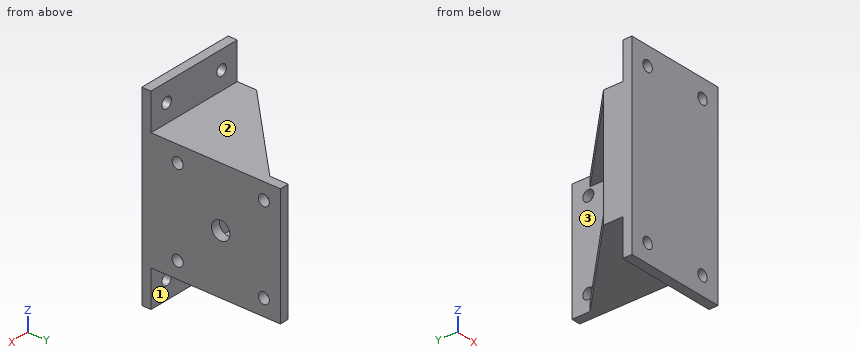
from build123d import *

# Parameters (mm, degrees)
BOSS_EXTRUDE1_DEPTH = 65
BOSS_EXTRUDE2_DEPTH = 5
BOSS_EXTRUDE3_DEPTH = 5
SKETCH4_R           = 5
SKETCH4_R_2         = 3
CUT_EXTRUDE1_DEPTH  = 102.612007165
SKETCH5_W           = 55
SKETCH5_H           = 20
BOSS_EXTRUDE4_DEPTH = 5
SKETCH6_R           = 3
CUT_EXTRUDE2_DEPTH  = 5


with BuildPart() as part:
    # Sketch1 → Boss-Extrude1 (new body)
    with BuildSketch(Plane.XY):
        Polygon((0, 0), (0, 60), (5, 60), (5, -15.5), (-50, -15.5), (-50, 0), align=None)
    extrude(amount=BOSS_EXTRUDE1_DEPTH)

    # Sketch2 → Boss-Extrude2 (add)
    with BuildSketch(Plane(origin=(0, 0, 0), x_dir=(-1, 0, 0), z_dir=(0, 0, -1))):
        Polygon((0, 0), (50, 0), (0, 50), align=None)
    extrude(amount=-BOSS_EXTRUDE2_DEPTH)

    # Sketch3 → Boss-Extrude3 (add)
    with BuildSketch(Plane.XY.offset(65)):
        Polygon((-50, 0), (0, 0), (0, 50), align=None)
    extrude(amount=-BOSS_EXTRUDE3_DEPTH)

    # Sketch4 → Cut-Extrude1 (cut, through all)
    with BuildSketch(Plane.ZY):
        with Locations(Location((32.5, 27.5, 0), (0, 0, 270))):
            Circle(SKETCH4_R)
        with Locations(Location((9, 51, 0), (0, 0, 270))):
            Circle(SKETCH4_R_2)
        with Locations(Location((56, 51, 0), (0, 0, 270))):
            Circle(SKETCH4_R_2)
        with Locations(Location((56, 4, 0), (0, 0, 270))):
            Circle(SKETCH4_R_2)
        with Locations(Location((9, 4, 0), (0, 0, 270))):
            Circle(SKETCH4_R_2)
    extrude(amount=-CUT_EXTRUDE1_DEPTH, mode=Mode.SUBTRACT)

    # Sketch5 → Boss-Extrude4 (add)
    with BuildSketch(Plane.XZ.offset(15.5)):
        with Locations((-22.5, -10)):
            Rectangle(SKETCH5_W, SKETCH5_H)
        with Locations((-22.5, 75)):
            Rectangle(SKETCH5_W, SKETCH5_H)
    extrude(amount=-BOSS_EXTRUDE4_DEPTH)

    # Sketch6 → Cut-Extrude2 (cut)
    with BuildSketch(Plane(origin=(0, -10.5, 0), x_dir=(1, 0, 0), z_dir=(0, 1, 0))):
        with Locations(Location((-5, 10, 0), (0, 0, 180))):
            Circle(SKETCH6_R)
        with Locations(Location((-40, 10, 0), (0, 0, 180))):
            Circle(SKETCH6_R)
        with Locations((-5, -75)):
            Circle(SKETCH6_R)
        with Locations((-40, -75)):
            Circle(SKETCH6_R)
    extrude(amount=-CUT_EXTRUDE2_DEPTH, mode=Mode.SUBTRACT)


solid = part.part
Model file for the job. Use its own axes, mm. Face numbers are marked on the shaded views. A direction names the side the tool comes from. Give positions to 0.01 mm unless a question says otherwise; leave off trailing zeros. Write each loop counter-clockwise with the first axis right and the second up, starting at its lowest first coordinate (ties: lowest second). Pieces come first, ordered by that corner, then holes. Notation, with made-up numbers: (10.25, 52) - (54.25, 52) arc R15 ccw to (54.25, 78) - close; hole circle Ø7 at (-35, -28). An arc over 180 degrees is marked (long way). Answer as CSV lines item,"result".
1. Pin check, flat tips, straight feed: pin 1 (25 mm diameter, centred on x = -19.5, y = 35.5, fed in from +Z); pin 2 (6 mm diameter, centred on x = -34.5, z = -9.5, fed in from +Y); pin 3 (6 mm diameter, centred on x = -38.5, z = 36.5, fed in from +Y). Stop position of each tip, or through.
Responses:
pin 1,"stops at z = 65"
pin 2,"stops at y = -10.5"
pin 3,"stops at y = 0"
2. Band-saw the part on D-D (y = 4). Write the cut outline in (x, z).
Responses:
outline,"(-46, 0) - (5, 0) - (5, 6) - (0, 6) - (0, 5) - (-46, 5) - close; (-46, 60) - (0, 60) - (0, 59) - (5, 59) - (5, 65) - (-46, 65) - close; (0, 12) - (5, 12) - (5, 53) - (0, 53) - close"
3. Band-saw the part on C-C (x = -11.5). Write the cut outline in (y, z).
Responses:
outline,"(-15.5, -20) - (-10.5, -20) - (-10.5, 0) - (38.5, 0) - (38.5, 5) - (0, 5) - (0, 60) - (38.5, 60) - (38.5, 65) - (-10.5, 65) - (-10.5, 85) - (-15.5, 85) - close"
4. Drill centre lines: L1, parallel to Z at x = -5, y = -13.45; L2, parallel to Z at x = 3, y = 4; L3, parallel to X at y = -12.05, z = 75. Where is each one in solid material? Low to high. Write a range as [from, to].
Responses:
L1,"z = [-20, -13], [-7, 72], [78, 85]"
L2,"z = [0, 6], [12, 53], [59, 65]"
L3,"x = [-50, -43], [-37, -8], [-2, 5]"
5. Band-saw the part on B-B (y = 27.5). Write the cut outline in (x, z), and give its area (3 significant figures).
Responses:
outline,"(-22.5, 0) - (5, 0) - (5, 27.5) - (0, 27.5) - (0, 5) - (-22.5, 5) - close; (-22.5, 60) - (0, 60) - (0, 37.5) - (5, 37.5) - (5, 65) - (-22.5, 65) - close"
area,"500 mm2"
6. Band-saw the part on A-A (z = 9). Write the cut outline in (x, y).
Responses:
outline,"(-50, -15.5) - (5, -15.5) - (5, 1) - (0, 1) - (0, 0) - (-50, 0) - close; (0, 7) - (5, 7) - (5, 48) - (0, 48) - close; (0, 54) - (5, 54) - (5, 60) - (0, 60) - close"
7. 3-axis set-ups, long thin cutter, end or side, ignore diameter. For the marked faces 1, 2 and 3: which of +Z, -Z, +X, -X, +Y, -Y reach the whole face in a straight line?
Responses:
face 1,"-Z, +X, -X, +Y"
face 2,"+Z, +X, -X, +Y"
face 3,"-X, +Y"
